Input: part model. Units: mm. Frame: model coordinates. A direction names the side the tool comes from. Round coordinates to 2 decimals unless told otherwise and drop trailing zeros. Loops run counter-clockwise (first coordinate to the right, second up) from the corner with the lowest first, then second, coordinate; pieces in that order, holes last. Notation, with made-up numbers: (19, 42) - (53, 42) arc R16 ccw to (53, 64) - close; hole circle Ø1 at (74.25, 75). An arc over 180 degrees is marked (long way). Write each question's results on one line, items separated by ' | '.
from build123d import *

# Parameters (mm, degrees)
PAD_DEPTH        = 22.6
THICKNESS_T      = 2.6
SKETCH001_W      = 57.4
SKETCH001_H      = 19.5
POCKET_DEPTH     = 5
SKETCH002_W      = 15.7
SKETCH002_H      = 20.5
POCKET001_DEPTH  = 5
HOLE_D           = 3.4
HOLE_DEPTH       = 25
HOLE_CBORE_D     = 6.1
HOLE_CBORE_DEPTH = 1.6
HOLE_TIPS_R      = 1.7


with BuildPart() as part:
    # Sketch → Pad (new body)
    with BuildSketch(Plane.XY):
        with BuildLine():
            ThreePointArc((-40.38, 15.5), (-41.278026, 15.128026), (-41.65, 14.23))
            Line((-41.65, -14.23), (-41.65, 14.23))
            ThreePointArc((-41.65, -14.23), (-41.278026, -15.128026), (-40.38, -15.5))
            Line((40.38, -15.5), (-40.38, -15.5))
            ThreePointArc((40.38, -15.5), (41.278026, -15.128026), (41.65, -14.23))
            Line((41.65, 14.23), (41.65, -14.23))
            ThreePointArc((41.65, 14.23), (41.278026, 15.128026), (40.38, 15.5))
            Line((-40.38, 15.5), (40.38, 15.5))
        make_face()
    extrude(amount=PAD_DEPTH)

    # Thickness
    thickness_openings = [part.faces().sort_by_distance(p)[0] for p in [
        (0, 0, 0),
    ]]
    offset(amount=THICKNESS_T, openings=thickness_openings)

    # Sketch001 → Pocket (cut)
    with BuildSketch(Plane.XZ.offset(18.1)):
        with Locations((5.15, 9.75)):
            Rectangle(SKETCH001_W, SKETCH001_H)
    extrude(amount=-POCKET_DEPTH, mode=Mode.SUBTRACT)

    # Sketch002 → Pocket001 (cut)
    with BuildSketch(Plane.YZ.offset(-44.25)):
        with Locations((0, 10.25)):
            Rectangle(SKETCH002_W, SKETCH002_H)
    extrude(amount=POCKET001_DEPTH, mode=Mode.SUBTRACT)

    # Hole
    with Locations(Plane.XY.offset(25.2)):
        with Locations((0, 4.592)):
            CounterBoreHole(HOLE_D / 2, HOLE_CBORE_D / 2, HOLE_CBORE_DEPTH, depth=HOLE_DEPTH)

    # Hole tips → Hole tip 1 section 0
    with BuildSketch(Plane.XY.offset(0.2), mode=Mode.PRIVATE) as hole_tip_1_s0:
        with Locations((0, 4.592)):
            Circle(HOLE_TIPS_R)
    loft([hole_tip_1_s0.sketch, Vertex(0, 4.592, -0.821463)], mode=Mode.SUBTRACT)


solid = part.part
1. Section query C-C, the plane x = 37.5. Output: boundary loops of the cut face in (y, z).
Answer:
outline: (-18.1, 0) - (-15.5, 0) - (-15.5, 22.6) - (15.5, 22.6) - (15.5, 0) - (18.1, 0) - (18.1, 22.6) arc R2.6 ccw to (15.5, 25.2) - (-15.5, 25.2) arc R2.6 ccw to (-18.1, 22.6) - close
2. Mould query, pull axis X, two halves, no side actions, for faces 4 (the cylindrical face through (-43.509, 0.199, 24.418)), 5 (the cylindrical face through (0.565, 17.359, 24.418)), 6 (the flat face through (-8, -15.5, 21)). Classes: pulls with the +X half, pulls with the -X half, needs draft (parallel to the pull), parting line crosses it, or undercut.
Answer:
face 4: pulls with the -X half | face 5: needs draft | face 6: undercut
3. Set-up query: faces 1 (the flat face through (33.85, -17, 10)), 2 (the flat face through (-43, 7.85, 10)), 3 (the flat face through (-1, 0, 22.6)). Return all of +Z, -Z, +X, -X, +Y, -Y with unobstructed straight access to the full face (end or side cutting, diameter ignored); none if empty.
Answer:
face 1: -Z, -Y | face 2: -Z, -X | face 3: -Z
4. Line query: line 1 (Y direction, x = -35.5, z = 22.5); line 2 (X direction, y = -12, z = 20.25); line 3 (Z direction, x = -4.5, y = -5). Output: solid intervals per line, ascending. Write a range as [from, to].
Answer:
line 1: [-18.1, -15.5], [15.5, 18.1] | line 2: [-44.25, -41.65], [41.65, 44.25] | line 3: [22.6, 25.2]
5. Contact query for flat-ended pins moving along their axis: pin 1 (0.8 mm diameter, centred on x = -43.5, y = 1, fed in from -Z); pin 2 (2 mm diameter, centred on y = 4, z = 17, fed in from -X); pin 3 (1.3 mm diameter, centred on x = 7, y = -17.5, fed in from -Z); pin 4 (1.8 mm diameter, centred on x = 0, y = 4, fed in from +Z). Output: stop coordinate, or through.
Answer:
pin 1: z = 20.5 | pin 2: x = 41.65 | pin 3: z = 19.5 | pin 4: through
6. Section query A-A, the plane x = 0. Output: boundary loops of the cut face in (y, z), plus the area to 3 significant figures.
Answer:
outline: (-18.1, 19.5) - (-15.5, 19.5) - (-15.5, 22.6) - (2.89, 22.6) - (2.89, 23.6) - (1.54, 23.6) - (1.54, 25.2) - (-15.5, 25.2) arc R2.6 ccw to (-18.1, 22.6) - close; (6.29, 22.6) - (15.5, 22.6) - (15.5, 0) - (18.1, 0) - (18.1, 22.6) arc R2.6 ccw to (15.5, 25.2) - (7.64, 25.2) - (7.64, 23.6) - (6.29, 23.6) - close | area: 145 mm^2
7. Section query B-B, the plane y = -3. Output: boundary loops of the cut face in (x, z), plus the area to 3 significant figures.
Answer:
outline: (-44.25, 20.5) - (-41.65, 20.5) - (-41.65, 22.6) - (41.65, 22.6) - (41.65, 0) - (44.25, 0) - (44.25, 22.6) arc R2.6 ccw to (41.65, 25.2) - (-41.65, 25.2) arc R2.6 ccw to (-44.25, 22.6) - close | area: 291 mm^2
